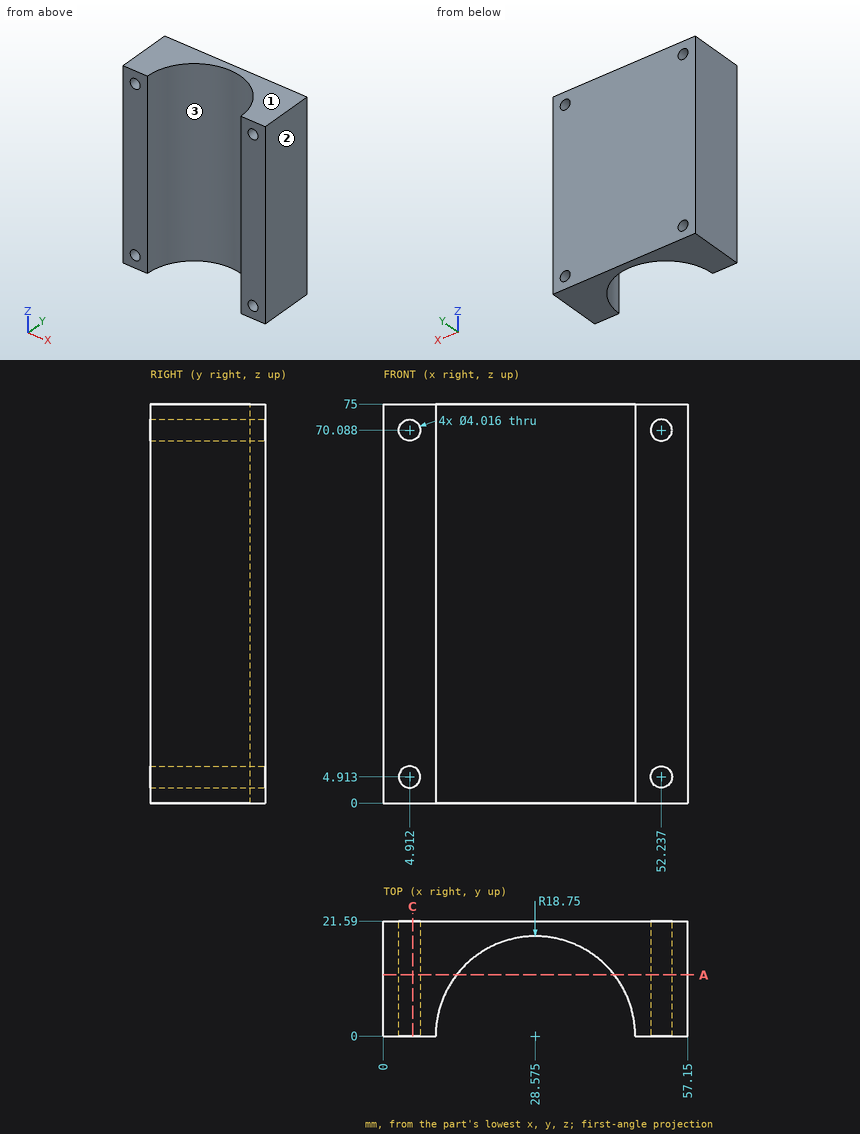
Here's the drawing with two shaded views (mm, measured from the low corner). I have some questions. Give positions to 0.01 mm unless a question says otherwise; leave off trailing zeros. Loops run counter-clockwise (first coordinate to the right, second up) from the corner with the lowest first, then second, coordinate; pieces in that order, holes last. Notation, with made-up numbers: M 82.25,72 L 88.25,72 A17 cw 88.25,95 Z; hole C 87,59 d10. An arc over 180 degrees is marked long. Use one line per item in the form item = value. Start each with the question number.
(1) Please list where these lines run through material, in increasing order: line 1 (X direction, y = 2, z = 14.5); line 2 (X direction, y = 5.75, z = 65); line 3 (Y direction, x = 42.5, z = 43) (1 decimal).
(2) I want a section at C-C, the plane x = 5.5. Write out the boundary of the cut face in (y, z), and give its area (3 significant figures).
(3) Thinking about a two-plate mould opening in X: for the marked faces 1, 2 and 3, which applies, released by +X, released by -X, zero draft, split by the parting line, or undercut?
(4) I want a section at A-A, the plane y = 11.5. State how many separate pieces and enclosed holes the cut face has, and give its area (3 significant figures).
(5) I'm going to push a flat-ended pin straight in: P1, Ø2.5, axis at x = 4.91, z = 70.09, coming from the -Y side. Where does the tip first touch, or does it pass through?
Worked out:
q1.line_1 = 0 to 9.93, 47.22 to 57.15
q1.line_2 = 0 to 10.73, 46.42 to 57.15
q1.line_3 = 12.6 to 21.6
q2.outline = M 0,0 L 21.59,0 L 21.59,2.99 L 0,2.99 Z; M 0,6.83 L 21.59,6.83 L 21.59,68.17 L 0,68.17 Z; M 0,72.01 L 21.59,72.01 L 21.59,75 L 0,75 Z
q2.area = 1,450 mm²
q3.face_1 = zero draft
q3.face_2 = released by +X
q3.face_3 = undercut
q4.separate_pieces = 2
q4.enclosed_holes = 4
q4.area = 2,010 mm²
q5.P1 = through
